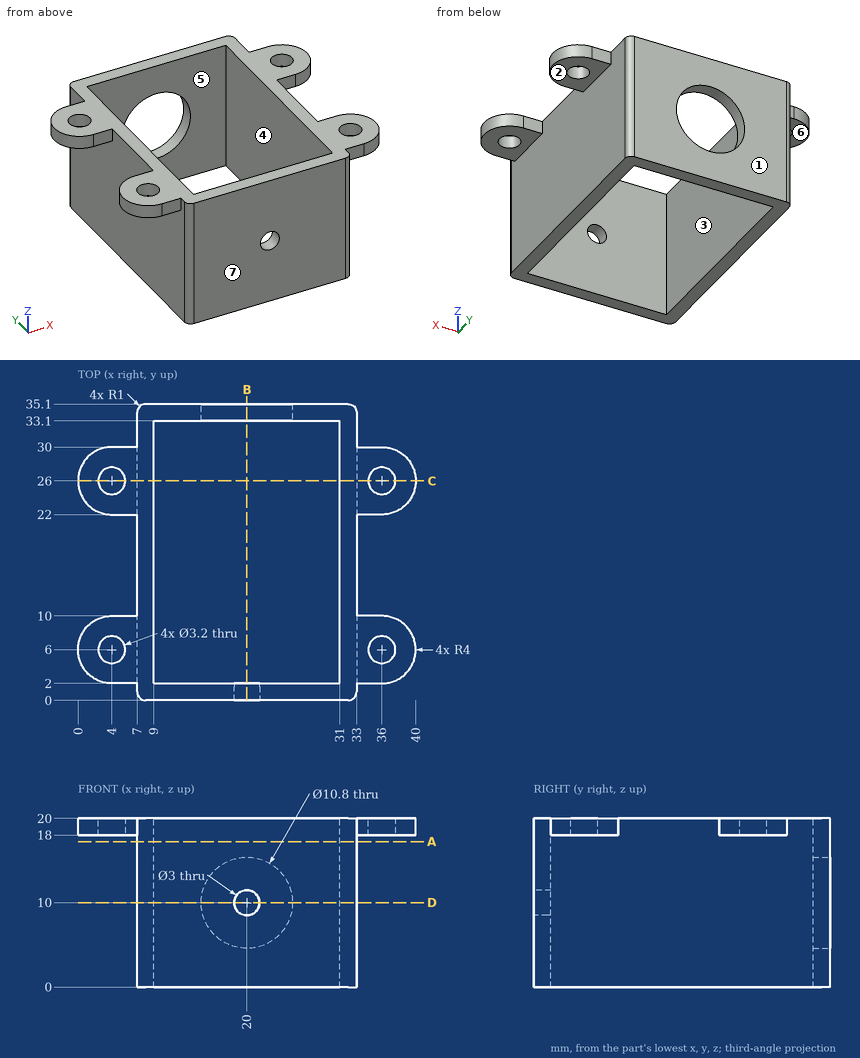
Check sheet for the drawn part. Datum: minimum x, y, z corner. Units: mm. A direction names the side the tool comes from. Round coordinates to 2 decimals unless told otherwise and drop trailing zeros. Order: outer loops, then holes, each group sorted by start corner. A loop starts at its lowest first (then second) coordinate and runs counter-clockwise, first axis right, second up. Notation, with made-up numbers: (9, -16.75) -> (30, -16.75) arc R19 ccw to (30, 8.25) -> close; hole circle Ø7 at (-31, 89). An arc over 180 degrees is marked (long way). Put each result on its own line as item: value.
1) Section check B-B (x = 20). Record the cut outline in (y, z), then the cut area to 3 significant figures.
Final values:
outline: (0, 0) -> (2, 0) -> (2, 8.5) -> (0, 8.5) -> close; (0, 11.5) -> (2, 11.5) -> (2, 20) -> (0, 20) -> close; (33.1, 0) -> (35.1, 0) -> (35.1, 4.6) -> (33.1, 4.6) -> close; (33.1, 15.4) -> (35.1, 15.4) -> (35.1, 20) -> (33.1, 20) -> close
area: 52.4 mm^2
2) Section check A-A (z = 17.25). Record the cut outline in (x, y).
Final values:
outline: (7, 1) arc R1 ccw to (8, 0) -> (32, 0) arc R1 ccw to (33, 1) -> (33, 34.1) arc R1 ccw to (32, 35.1) -> (8, 35.1) arc R1 ccw to (7, 34.1) -> close; hole (9, 2) -> (31, 2) -> (31, 33.1) -> (9, 33.1) -> close
3) Depth check by flat-ended pin: pin 1 (10 mm diameter, centred on y = 15, z = 14.5, fed in from -X); pin 2 (10 mm diameter, centred on y = 17, z = 6.5, fed in from +X); pin 3 (3.5 mm diameter, centred on x = 5, y = 5.5, fed in from -Z). Enter the tip coordinate at first touch or a pass-through.
Final values:
pin 1: stops at x = 7
pin 2: stops at x = 33
pin 3: stops at z = 18
4) Material ranges on line 1 (Y direction, x = 36, z = 19.2); line 2 (Y direction, x = 13, z = 4.5); line 3 (X direction, y = 1, z = 10), recorded low to high.
Final values:
line 1: y = 2 to 4.4, 7.6 to 10, 22 to 24.4, 27.6 to 30
line 2: y = 0 to 2, 33.1 to 35.1
line 3: x = 7 to 18.5, 21.5 to 33
5) Section check D-D (z = 10). Record the cut outline in (x, y), then the cut area to 3 significant figures.
Final values:
outline: (7, 1) arc R1 ccw to (8, 0) -> (18.5, 0) -> (18.5, 2) -> (9, 2) -> (9, 33.1) -> (14.6, 33.1) -> (14.6, 35.1) -> (8, 35.1) arc R1 ccw to (7, 34.1) -> close; (21.5, 0) -> (32, 0) arc R1 ccw to (33, 1) -> (33, 34.1) arc R1 ccw to (32, 35.1) -> (25.4, 35.1) -> (25.4, 33.1) -> (31, 33.1) -> (31, 2) -> (21.5, 2) -> close
area: 200 mm^2
6) Section check C-C (y = 26). Record the cut outline in (x, z), then the cut area to 3 significant figures.
Final values:
outline: (0, 18) -> (2.4, 18) -> (2.4, 20) -> (0, 20) -> close; (5.6, 18) -> (7, 18) -> (7, 0) -> (9, 0) -> (9, 20) -> (5.6, 20) -> close; (31, 0) -> (33, 0) -> (33, 18) -> (34.4, 18) -> (34.4, 20) -> (31, 20) -> close; (37.6, 18) -> (40, 18) -> (40, 20) -> (37.6, 20) -> close
area: 95.2 mm^2
7) Mould release check, pull along Y, two halves, no side actions. Record for the marked faces 4, 5, 6 and 7: +Y half, -Y half, draft (parallel to the pull), parting line (faces both ways), or undercut.
Final values:
face 4: undercut
face 5: undercut
face 6: draft
face 7: -Y half
8) Set-up check for the marked faces 1, 2 and 3: record each of +Z, -Z, +X, -X, +Y, -Y from which the full face is reachable in a straight line by a thin tool's end or side.
Final values:
face 1: +Z, -Z, +X, -X, +Y
face 2: -Z, +X, +Y, -Y
face 3: +Z, -Z
